Source: CAD feature listing. Evaluate the final solid. Frame: model axes, mm. A direction names the side the tool comes from. Give positions to 0.01 mm unless a question says otherwise; leave off trailing zeros. Loops run counter-clockwise (first coordinate to the right, second up) from the corner with the lowest first, then second, coordinate; pieces in that order, holes last. Notation, with made-up numbers: M 64,49.5 L 123,49.5 A22 ccw 123,74.5 Z; hole C 43.25,4.25 d4. An arc over 180 degrees is marked long. Answer in a Markdown table with one row per item.
Autodesk Inventor part; units mm, degrees
ref_plane "YZ Plane" through (0, 0, 0) normal (1, 0, 0) x (0, 1, 0)
ref_plane "XZ Plane" through (0, 0, 0) normal (0, 1, 0) x (-1, 0, 0)
ref_plane "XY Plane" through (0, 0, 0) normal (0, 0, 1) x (1, 0, 0)
sketch "Esquisse1" plane through (0, 0, 0) normal (0, 1, 0) x (-1, 0, 0)
  line L0 (0, 0) -> (-15, 0)
  line L1 (-15, 0) -> (-15, -15)
  line L2 (-15, -15) -> (0, -15)
  line L3 (0, -15) -> (0, 0)
  dimension "d0" = 15
  dimension "d1" = 15
extrude "Extrusion1" add sketch "Esquisse1" along normal blind 10
sketch "Esquisse2" plane through (0, 10, 0) normal (0, 1, 0) x (1, 0, 0)
  line L0 (0, 15) -> (0, 0)
  line L1 (0, 8.6556) -> (15, 8.6556)
  line L2 (15, 8.6556) -> (15, 23.6556)
  line L3 (15, 23.6556) -> (0, 23.6556)
  line L4 (0, 23.6556) -> (0, 8.6556)
  dimension "d4" = 15
  dimension "d5" = 15
extrude "Extrusion2" add sketch "Esquisse2" along normal blind 10
1) Set-up query: faces 4 (the flat face through (8, 5, -15)), 5 (the flat face through (8, 10, -4)), 6 (the flat face through (15, 10, -12)). Return all of +Z, -Z, +X, -X, +Y, -Y with unobstructed straight access to the full face (end or side cutting, diameter ignored); none if empty.
Reply:
| item | result |
|---|---|
| face 4 | -Z, +X, -X, -Y |
| face 5 | +Z, +X, -X, +Y |
| face 6 | +Z, -Z, +X, +Y, -Y |
2) Section C-C, the plane y = 17. Return loops of the section in (x, z).
Reply:
| item | result |
|---|---|
| outline | M 0,-23.66 L 15,-23.66 L 15,-8.66 L 0,-8.66 Z |
3) Material intervals for L1, parallel to Z at x = 9, y = 7.75; L2, parallel to Y at x = 7, z = -17.25; L3, parallel to Z at x = 13.5, y = 15.5, sorted ascending.
Reply:
| item | result |
|---|---|
| L1 | z = -15 to 0 |
| L2 | y = 10 to 20 |
| L3 | z = -23.66 to -8.66 |
4) Pin query (flat end, axial travel): pin 1 Ø3 at (x, y) = (10.5, 2.5) entering from -Z; pin 2 Ø7 at (x, z) = (10, -3) entering from +Y; pin 3 Ø1 at (x, z) = (4, -17) entering from -Y. Return the tip coordinate at first contact, or that it passes through.
Reply:
| item | result |
|---|---|
| pin 1 | stops at z = -15 |
| pin 2 | stops at y = 10 |
| pin 3 | stops at y = 10 |
5) Pull-direction query (Y, two-part tool) for faces 1 (the flat face through (7, 20, -16)), 2 (the flat face through (8, 0, -7)), 3 (the flat face through (7, 15, -8.656)); classes: released by +Y, released by -Y, zero draft, split by the parting line, or undercut.
Reply:
| item | result |
|---|---|
| face 1 | released by +Y |
| face 2 | released by -Y |
| face 3 | zero draft |
6) Section A-A, the plane x = 12.75. Return loops of the section in (y, z), then the cut area to 3 significant figures.
Reply:
| item | result |
|---|---|
| outline | M 0,-15 L 10,-15 L 10,-23.66 L 20,-23.66 L 20,-8.66 L 10,-8.66 L 10,0 L 0,0 Z |
| area | 300 mm² |
7) Section B-B, the plane z = -4.5. Return loops of the section in (x, y).
Reply:
| item | result |
|---|---|
| outline | M 0,0 L 15,0 L 15,10 L 0,10 Z |
